Part model, mm, in its own coordinate system. A direction names the side the tool comes from. Give positions to 0.01 mm unless a question says otherwise; leave off trailing zeros. Write each loop counter-clockwise with the first axis right and the second up, starting at its lowest first coordinate (ties: lowest second). Pieces come first, ordered by that corner, then holes.
```python
from build123d import *

# Parameters (mm, degrees)
M5X0_8_TAPPED_HOLE1_D     = 4.2
M5X0_8_TAPPED_HOLE1_DEPTH = 17.399
M5X0_8_TAPPED_HOLE1_TIP   = 1.2618073
CUT_EXTRUDE1_REACH        = 185.602
SKETCH7_W                 = 50.8
SKETCH7_H                 = 2.565921067
F_8_32_TAPPED_HOLE1_D     = 3.4544


with BuildPart() as part:
    # Sketch1 → Revolve1 (revolve)
    with BuildSketch(Plane.XY, mode=Mode.PRIVATE) as revolve1_sk:
        Polygon((80.3783, 0), (99.4283, 0), (99.4283, -6.985), (109.7915, -6.985), (109.7915, -9.525), (127, -9.525), (127, 28.575), (96.5, 28.575), (96.5, 8.255), (80.3783, 8.255), align=None)
    revolve(revolve1_sk.sketch.rotate(Axis((0, 0, 0), (0, 1, 0)), 90), axis=Axis((0, 0, 0), (0, 1, 0)))

    # M5x0.8 Tapped Hole1
    with Locations(Plane(origin=(0, 28.575, 0), x_dir=(1, 0, 0), z_dir=(0, 1, 0))):
        with Locations((0, 102.5), (72.478445072, 72.478445072), (102.5, 0), (72.478445072, -72.478445072), (0, -102.5), (-72.478445072, -72.478445072), (-102.5, 0), (-72.478445072, 72.478445072)):
            Hole(M5X0_8_TAPPED_HOLE1_D / 2, depth=M5X0_8_TAPPED_HOLE1_DEPTH)
            with Locations((0, 0, -(M5X0_8_TAPPED_HOLE1_DEPTH + M5X0_8_TAPPED_HOLE1_TIP / 2))):  # 118° drill point
                Cone(0, M5X0_8_TAPPED_HOLE1_D / 2, M5X0_8_TAPPED_HOLE1_TIP, mode=Mode.SUBTRACT)

    # Sketch7 → Cut-Extrude1 (cut, up to next)
    with BuildSketch(Plane(origin=(0, 28.575, 0), x_dir=(1, 0, 0), z_dir=(0, 1, 0)), mode=Mode.PRIVATE) as cut_extrude1_sk1:
        with Locations((0, -125.717039467)):
            Rectangle(SKETCH7_W, SKETCH7_H)
    cut_extrude1_tool1 = extrude(cut_extrude1_sk1.sketch, amount=-CUT_EXTRUDE1_REACH, mode=Mode.PRIVATE) & part.part
    add(cut_extrude1_tool1.solids().sort_by_distance((0, 28.575, 125.717039))[0], mode=Mode.SUBTRACT)

    # #8-32 Tapped Hole1 (through all)
    with Locations(Plane(origin=(0, 0, 0), x_dir=(-1, 0, 0), z_dir=(0, -1, 0))):
        with Locations((-6.35, -85.09), (6.35, -85.09)):
            Hole(F_8_32_TAPPED_HOLE1_D / 2)


solid = part.part
```
1) 3-axis set-ups, long thin cutter, end or side, ignore diameter. For faces 5 (the face through (0, 0, 81)), 6 (the face through (-28.986, 18.273, -92.044)), 7 (the face through (0, 10, 124.434)): which of +Z, -Z, +X, -X, +Y, -Y reach the whole face in a straight line?
Answers follow:
face 5: -Y
face 6: +Y
face 7: +Z, +X, -X, +Y, -Y
2) Saw through at B-B, the plane x = 20.5. Write the cut outline in (y, z) (3 decimals).
Answers follow:
outline: (-9.525, -125.335) - (28.575, -125.335) - (28.575, -94.297) - (8.255, -94.297) - (8.255, -77.72) - (0, -77.72) - (0, -97.292) - (-6.985, -97.292) - (-6.985, -107.861) - (-9.525, -107.861) - close; (-9.525, 107.861) - (-6.985, 107.861) - (-6.985, 97.292) - (0, 97.292) - (0, 77.72) - (8.255, 77.72) - (8.255, 94.297) - (28.575, 94.297) - (28.575, 124.434) - (-9.525, 124.434) - close
3) Two-plate mould, pull along X, no slides. Class faces 1 (the face through (5.226, 9.792, -126.892)), 2 (the face through (48.909, 4.07, 63.785)), 3 (the face through (-82, -6.985, -57)), 4 (the face through (103, -9.525, -39)): +X half, -X half, draft (parallel to the pull), parting line (faces both ways), or undercut.
Answers follow:
face 1: parting line
face 2: undercut
face 3: undercut
face 4: draft
4) Saw through at C-C, the plane y = 23.5. Count the separate pieces of the cut face and the enclosed holes in it, then the cut area to 3 significant figures.
Answers follow:
separate pieces: 1
enclosed holes: 9
area: 21,200 mm2
5) Pin check, flat tips, straight feed: pin 1 Ø5.5 at (x, z) = (0, 102.5) entering from +Y (3 decimals); pin 2 Ø5 at (y, z) = (4.5, -99) entering from -X; pin 3 Ø3 at (x, z) = (6.35, 85.09) entering from -Y; pin 4 Ø4 at (x, y) = (91, 13.5) entering from +Z. Stop position of each tip, or through.
Answers follow:
pin 1: stops at y = 28.575
pin 2: stops at x = -82.56
pin 3: passes through
pin 4: stops at z = 90.6
6) Wall check: L1, parallel to X at y = -5, z = 0; L2, parallel to X at y = 6, z = 85; L3, parallel to X at y = -8.6, z = 0. Give the ranges that are in metal, low to high.
Answers follow:
L1: x = -127 to -99.43, 99.43 to 127
L2: x = -94.36 to -8.07, -4.63 to 4.63, 8.07 to 94.36
L3: x = -127 to -109.79, 109.79 to 127
7) Saw through at A-A, the plane z = -34. Write the cut outline in (x, y) (3 decimals).
Answers follow:
outline: (-122.364, -9.525) - (-104.394, -9.525) - (-104.394, -6.985) - (-93.434, -6.985) - (-93.434, 0) - (-72.833, 0) - (-72.833, 8.255) - (-90.312, 8.255) - (-90.312, 28.575) - (-122.364, 28.575) - close; (72.833, 0) - (93.434, 0) - (93.434, -6.985) - (104.394, -6.985) - (104.394, -9.525) - (122.364, -9.525) - (122.364, 28.575) - (90.312, 28.575) - (90.312, 8.255) - (72.833, 8.255) - close
